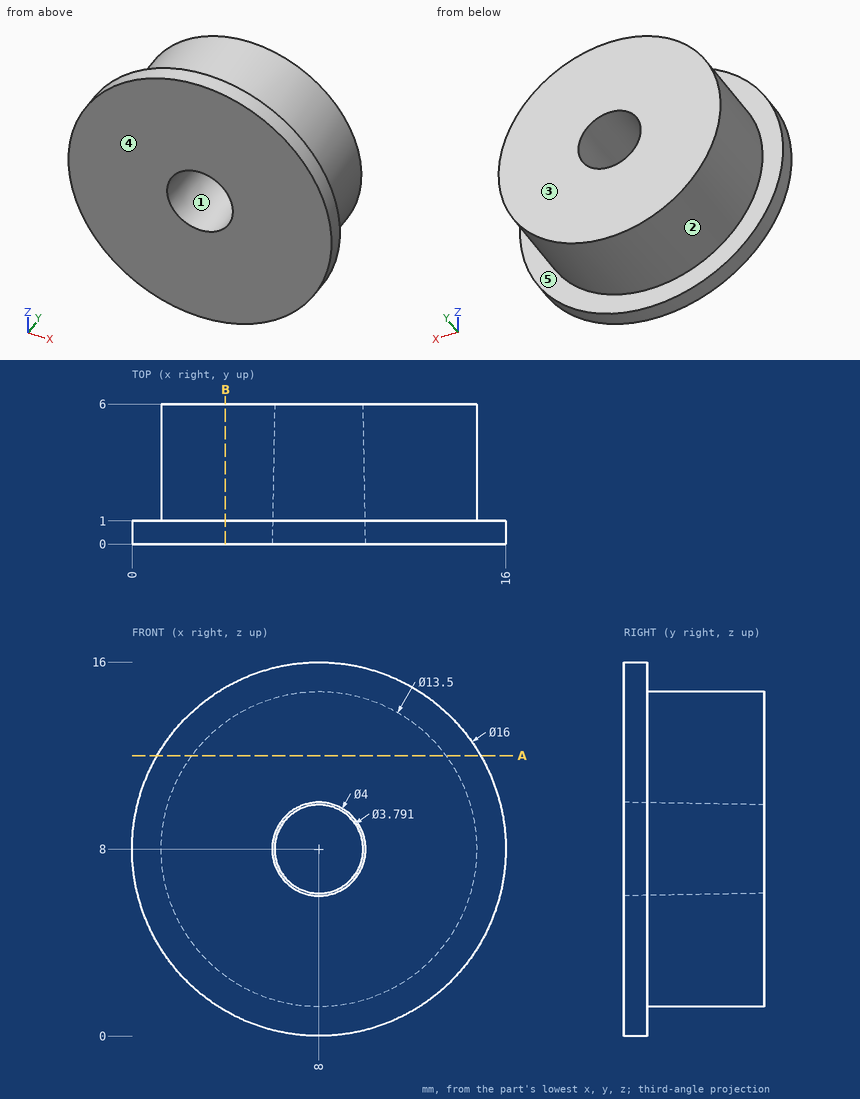
Input: dimensioned drawing with shaded views. Units: mm. Origin: part minimum x, y, z. A direction names the side the tool comes from. Coordinates: 2 decimals unless noted, no trailing zeros. Loops run counter-clockwise (first coordinate to the right, second up) from the corner with the lowest first, then second, coordinate; pieces in that order, holes last.
Q1. Mould query, pull axis Z, two halves, no side actions, for the marked faces 1, 2 and 3. Classes: +Z half, -Z half, draft (parallel to the pull), parting line (faces both ways), or undercut.
Results are:
face 1: undercut
face 2: parting line
face 3: draft
Q2. Set-up query: the marked faces 4 and 5. Return all of +Z, -Z, +X, -X, +Y, -Y with unobstructed straight access to the full face (end or side cutting, diameter ignored); none if empty.
Results are:
face 4: +Z, -Z, +X, -X, -Y
face 5: +Y
Q3. Section A-A, the plane z = 12. Return the cut outline in (x, y).
Results are:
outline: (1.07, 0) - (14.93, 0) - (14.93, 1) - (13.44, 1) - (13.44, 6) - (2.56, 6) - (2.56, 1) - (1.07, 1) - close
Q4. Contact query for flat-ended pins moving along their axis: pin 1 (1 mm diameter, centred on y = 3, z = 12.5, fed in from -X); pin 2 (3 mm diameter, centred on y = 4.5, z = 8.5, fed in from -X); pin 3 (1 mm diameter, centred on y = 2.5, z = 12, fed in from +X). Output: stop coordinate, or through.
Results are:
pin 1: stops at x = 2.56
pin 2: stops at x = 1.25
pin 3: stops at x = 13.77
Q5. Line query: line 1 along X through (y, z) = (5.5, 8.5); line 2 along Y through (x, z) = (2, 12.75); line 3 along X through (y, z) = (4, 6.75) (1 decimal). Output: solid intervals per line, ascending.
Results are:
line 1: x = 1.27 to 6.16, 9.84 to 14.73
line 2: y = 0 to 1
line 3: x = 1.4 to 6.5, 9.5 to 14.6
Q6. Section B-B, the plane x = 4. Return the cut outline in (y, z).
Results are:
outline: (0, 1.07) - (1, 1.07) - (1, 2.56) - (6, 2.56) - (6, 13.44) - (1, 13.44) - (1, 14.93) - (0, 14.93) - close
